from build123d import *

# Parameters (mm, degrees)
SKETCH1_W                = 300
SKETCH1_H                = 2000
BOSS_EXTRUDE1_DEPTH      = 10
BOSS_EXTRUDE2_START      = 80
BOSS_EXTRUDE2_DEPTH      = 60
BOSS_EXTRUDE3_START      = -140
BOSS_EXTRUDE3_DEPTH      = 60
BOSS_EXTRUDE4_DEPTH      = 150
BOSS_EXTRUDE4_DEPTH_BACK = 150


with BuildPart() as part:
    # Sketch1 → Boss-Extrude1 (new body)
    with BuildSketch(Plane(origin=(0, 0, 0), x_dir=(1, 0, 0), z_dir=(0, 1, 0))):
        Rectangle(SKETCH1_W, SKETCH1_H)
    extrude(amount=BOSS_EXTRUDE1_DEPTH)

    # Sketch2 → Boss-Extrude2 (add)
    with BuildSketch(Plane(origin=(0, 0, 0), x_dir=(0, 0, -1), z_dir=(1, 0, 0)).offset(BOSS_EXTRUDE2_START)):
        Polygon((530, 10), (554.216468309, 35), (575.783531691, 35), (600, 10), align=None)
    extrude(amount=BOSS_EXTRUDE2_DEPTH)

    # Sketch3 → Boss-Extrude3 (add)
    with BuildSketch(Plane(origin=(0, 0, 0), x_dir=(0, 0, -1), z_dir=(1, 0, 0)).offset(BOSS_EXTRUDE3_START)):
        Polygon((60, 10), (79.278295144, 35), (110.721704856, 35), (130, 10), align=None)
    extrude(amount=BOSS_EXTRUDE3_DEPTH)

    # Sketch4 → Boss-Extrude4 (add, two sides: drawn at the far end of the back side and taken through both)
    with BuildSketch(Plane(origin=(0, 0, 0), x_dir=(0, 0, -1), z_dir=(1, 0, 0)).offset(-BOSS_EXTRUDE4_DEPTH_BACK)):
        Polygon((-410, 10), (-384.771871556, 35), (-365.228128444, 35), (-340, 10), align=None)
    extrude(amount=BOSS_EXTRUDE4_DEPTH + BOSS_EXTRUDE4_DEPTH_BACK)


solid = part.part
Geometry: final body of the model. Coordinates: model frame, mm. A direction names the side the tool comes from. Coordinates: 2 decimals unless noted, no trailing zeros. Loops run counter-clockwise (first coordinate to the right, second up) from the corner with the lowest first, then second, coordinate; pieces in that order, holes last. Notation, with made-up numbers: (-34, -38) - (-20, -38) arc R22 ccw to (-20, -25) - close; hole circle Ø5 at (79.5, 19.25). An arc over 180 degrees is marked (long way). Put each result on its own line as item: value. Start each with the question number.
Q1. Pin query (flat end, axial travel): pin 1 Ø8 at (x, z) = (26, 307) entering from -Y; pin 2 Ø7.5 at (y, z) = (25.5, -86.5) entering from +X; pin 3 Ø20 at (y, z) = (26.5, -548.5) entering from -X; pin 4 Ø5 at (x, y) = (69.5, 15) entering from +Z. Return the tip coordinate at first contact, or that it passes through.
Q2. Line query: line 1 (Y direction, x = -130, z = -671.5); line 2 (Z direction, x = -136.5, y = 18.5); line 3 (Z direction, x = -112.5, y = 22). Output: solid intervals per line, ascending.
Q3. Cut plane A-A, the plane y = 20.5. Return loops of the section in (x, z).
Q4. Pull-direction query (Z, two-part tool) for faces 3 (the flat face through (-2, 0, -14)), 4 (the flat face through (-2, 10, -339)); classes: released by +Z, released by -Z, zero draft, split by the parting line, or undercut.
Q5. Set-up query: faces 1 (the flat face through (-150, 6, 5)), 2 (the flat face through (-2, 10, 701)). Return all of +Z, -Z, +X, -X, +Y, -Y with unobstructed straight access to the full face (end or side cutting, diameter ignored); none if empty.
Q6. Cut plane C-C, the plane z = 112. Return loops of the section in (x, y), and give its area (3 significant figures).
Q7. Cut plane B-B, the plane x = 120. Return loops of the section in (y, z), and give its area (3 significant figures).
Q8. Cut plane D-D, the plane x = -40. Return loops of the section in (y, z).
Filled sheet:
1. pin 1: y = 0
1. pin 2: x = -80
1. pin 3: x = 80
1. pin 4: z = 407.48
2. line 1: 0 to 10
2. line 2: -123.45 to -66.55, 348.58 to 401.42
2. line 3: -120.75 to -69.25, 352.11 to 397.89
3. outline: (-150, 350.6) - (150, 350.6) - (150, 399.4) - (-150, 399.4) - close; (-140, -121.9) - (-80, -121.9) - (-80, -68.1) - (-140, -68.1) - close; (80, -589.83) - (140, -589.83) - (140, -540.17) - (80, -540.17) - close
4. face 3: zero draft
4. face 4: undercut
5. face 1: +Z, -Z, -X, +Y, -Y
5. face 2: +Z, +X, -X, +Y
6. outline: (-150, 0) - (150, 0) - (150, 10) - (-150, 10) - close
6. area: 3,000 mm²
7. outline: (0, -1000) - (10, -1000) - (10, -600) - (35, -575.78) - (35, -554.22) - (10, -530) - (10, 340) - (35, 365.23) - (35, 384.77) - (10, 410) - (10, 1000) - (0, 1000) - close
7. area: 22,300 mm²
8. outline: (0, -1000) - (10, -1000) - (10, 340) - (35, 365.23) - (35, 384.77) - (10, 410) - (10, 1000) - (0, 1000) - close
